from build123d import *

# Parameters (mm, degrees)
F1_DEPTH = 1
F2_R     = 3.25
F3_DEPTH = 5


with BuildPart() as f1:
    # F0 (on Top) → F1 (new body)
    with BuildSketch(Plane.XY):
        with BuildLine():
            Line((12.5, 15), (-12.5, 15))
            ThreePointArc((-12.5, 15), (-27.5, 0), (-12.5, -15))
            Line((-12.5, -15), (12.5, -15))
            ThreePointArc((12.5, -15), (27.5, 0), (12.5, 15))
        make_face()
    extrude(amount=F1_DEPTH)

    # F2 (on face) → F3 (join)
    with BuildSketch(Plane.XY.offset(1)):
        with Locations((-18.75, 0)):
            Circle(F2_R)
        with Locations((18.75, 0)):
            Circle(F2_R)
    extrude(amount=F3_DEPTH)


solid = f1.part
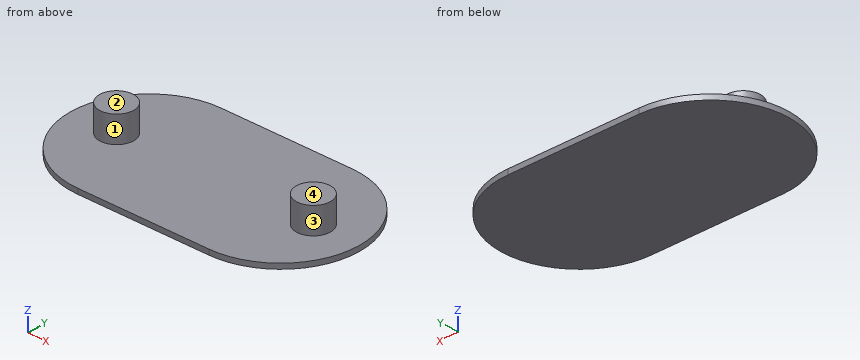
Design review of the part built by this model. Coordinates are the model's own, in mm. Face numbers are marked on the shaded views. A direction names the side the tool comes from. Coordinates: 2 decimals unless noted, no trailing zeros. Loops run counter-clockwise (first coordinate to the right, second up) from the corner with the lowest first, then second, coordinate; pieces in that order, holes last. Notation, with made-up numbers: M 60.25,61 L 81.25,61 A28 cw 81.25,83 Z; hole C -1.75,60.5 d6. An arc over 180 degrees is marked long. Use one line per item in the form item = value.
(1) Consider section B-B (z = 4.4). Write out the cut boundary in (x, y), and give its area (3 significant figures).
Return value:
outline = C -18.75,0 d6.5; C 18.75,0 d6.5
area = 66.4 mm2
(2) Consider section D-D (x = 18.5). Write out the cut boundary in (y, z).
Return value:
outline = M -13.75,0 L 13.75,0 L 13.75,1 L 3.24,1 L 3.24,6 L -3.24,6 L -3.24,1 L -13.75,1 Z
(3) For line 1 along Z through (x, y) = (-9.5, 2.5); line 2 along X through (y, z) = (-2, 1.1); line 3 along X through (y, z) = (3, 5.65), list the stretches that pass through material, from the lowest coordinate up. Write a range as from..to.
Return value:
line_1 = 0..1
line_2 = -21.31..-16.19, 16.19..21.31
line_3 = -20..-17.5, 17.5..20
(4) For the marked faces 3 and 4, list the 3-axis set-ups (+Z, -Z, +X, -X, +Y, -Y) from which the entire face can be reached by the end or side of a thin tool; tool diameter is ignored.
Return value:
face_3 = +Z
face_4 = +Z, +X, -X, +Y, -Y
(5) Consider section C-C (x = -8.5). Write out the cut boundary in (y, z), and give its area (3 significant figures).
Return value:
outline = M -15,0 L 15,0 L 15,1 L -15,1 Z
area = 30.0 mm2
(6) Draft analysis for pull direction X (two halves, no side actions). For the marked faces 1 and 2, state which applies: pulls with the +X half, pulls with the -X half, needs draft (parallel to the pull), parting line crosses it, or undercut.
Return value:
face_1 = undercut
face_2 = needs draft
(7) Clearance check with flat-ended pins moving along their axes: P1, Ø1.5, axis at x = 16, z = 3, coming from the +Y side; P2, Ø6, axis at x = 4.5, y = 2, coming from the +Z side. State where each tip first meets the part, or that it passes through.
Return value:
P1 = 2.56
P2 = 1
(8) Consider section A-A (y = 0). Write out the cut boundary in (x, z).
Return value:
outline = M -27.5,0 L 27.5,0 L 27.5,1 L 22,1 L 22,6 L 15.5,6 L 15.5,1 L -15.5,1 L -15.5,6 L -22,6 L -22,1 L -27.5,1 Z
